Design review of the part built by this model. Coordinates are the model's own, in mm. Coordinates: 2 decimals unless noted, no trailing zeros. Order: outer loops, then holes, each group sorted by start corner. A loop starts at its lowest first (then second) coordinate and runs counter-clockwise, first axis right, second up. Notation, with made-up numbers: M 50,83 L 63,83 A21 cw 63,97 Z; hole C 81.5,-37 d8. An arc over 180 degrees is marked long. Answer as a JSON object with one key per item and string values.
Autodesk Inventor part; units mm, degrees
ref_plane "YZ Plane" through (0, 0, 0) normal (1, 0, 0) x (0, 1, 0)
ref_plane "XZ Plane" through (0, 0, 0) normal (0, 1, 0) x (-1, 0, 0)
ref_plane "XY Plane" through (0, 0, 0) normal (0, 0, 1) x (1, 0, 0)
sketch "Sketch1" plane through (0, 0, 0) normal (1, 0, 0) x (0, 1, 0)
  line L0 (4.9868, 295.4813) -> (-299.8132, 295.4813)
  line L1 (-299.8132, 295.4813) -> (-299.8132, -9.3187)
  line L2 (-299.8132, -9.3187) -> (4.9868, -9.3187)
  line L3 (4.9868, -9.3187) -> (4.9868, 295.4813)
  point P0 (0, 0)
  dimension "d0" = 304.8
  dimension "d1" = 304.8
extrude "Extrusion1" add sketch "Sketch1" along normal blind 3.175
sketch "Sketch2" plane through (3.175, 0, 0) normal (1, 0, 0) x (0, 0, -1)
  line L0 (-143.0813, 4.9868) -> (-143.0813, -147.4132)
  circle A0 centre (-143.0813, -147.4132) radius 12.7
  point P0 (0, 0)
  point P1 (9.3187, 4.9868)
  dimension "d4" = 152.4
  dimension "d5" = 25.4
extrude "Extrusion2" cut sketch "Sketch2" against normal blind 50.8
sketch "Sketch3" plane through (3.175, 0, 0) normal (1, 0, 0) x (0, 0, -1)
  circle A0 centre (-143.0813, -147.4132) radius 12.7
  circle A1 centre (-143.0813, -122.0132) radius 3.175
  circle A2 centre (-143.0813, -96.6132) radius 3.175
  circle A3 centre (-143.0813, -71.2132) radius 3.175
  circle A4 centre (-143.0813, -45.8132) radius 3.175
  circle A5 centre (-143.0813, -20.4132) radius 3.175
  circle A6 centre (-143.0813, 4.9868) radius 3.175
  line L0 (9.3187, -299.8132) -> (9.3187, 4.9868)
  circle A7 centre (-143.0813, -172.8132) radius 3.175
  circle A8 centre (-143.0813, -198.2132) radius 3.175
  circle A9 centre (-143.0813, -249.0132) radius 3.175
  circle A10 centre (-143.0813, -223.6132) radius 3.175
  circle A11 centre (-143.0813, -299.8132) radius 3.175
  circle A12 centre (-143.0813, -274.4132) radius 3.175
  circle A13 centre (-168.4813, -122.0132) radius 3.175
  circle A14 centre (-168.4813, -96.6132) radius 3.175
  circle A15 centre (-168.4813, -45.8132) radius 3.175
  circle A16 centre (-168.4813, -71.2132) radius 3.175
  circle A17 centre (-168.4813, 4.9868) radius 3.175
  circle A18 centre (-168.4813, -20.4132) radius 3.175
  circle A19 centre (-168.4813, -299.8132) radius 3.175
  circle A20 centre (-168.4813, -249.0132) radius 3.175
  circle A21 centre (-168.4813, -274.4132) radius 3.175
  circle A22 centre (-168.4813, -223.6132) radius 3.175
  circle A23 centre (-168.4813, -198.2132) radius 3.175
  circle A24 centre (-168.4813, -172.8132) radius 3.175
  circle A25 centre (-117.6813, -122.0132) radius 3.175
  circle A26 centre (-117.6813, -96.6132) radius 3.175
  circle A27 centre (-117.6813, -45.8132) radius 3.175
  circle A28 centre (-117.6813, -71.2132) radius 3.175
  circle A29 centre (-117.6813, 4.9868) radius 3.175
  circle A30 centre (-117.6813, -20.4132) radius 3.175
  circle A31 centre (-117.6813, -299.8132) radius 3.175
  circle A32 centre (-117.6813, -249.0132) radius 3.175
  circle A33 centre (-117.6813, -274.4132) radius 3.175
  circle A34 centre (-117.6813, -223.6132) radius 3.175
  circle A35 centre (-117.6813, -198.2132) radius 3.175
  circle A36 centre (-117.6813, -172.8132) radius 3.175
  circle A37 centre (-193.8813, -122.0132) radius 3.175
  circle A38 centre (-193.8813, -96.6132) radius 3.175
  circle A39 centre (-193.8813, -45.8132) radius 3.175
  circle A40 centre (-193.8813, -71.2132) radius 3.175
  circle A41 centre (-193.8813, 4.9868) radius 3.175
  circle A42 centre (-193.8813, -20.4132) radius 3.175
  circle A43 centre (-193.8813, -299.8132) radius 3.175
  circle A44 centre (-193.8813, -249.0132) radius 3.175
  circle A45 centre (-193.8813, -274.4132) radius 3.175
  circle A46 centre (-193.8813, -223.6132) radius 3.175
  circle A47 centre (-193.8813, -198.2132) radius 3.175
  circle A48 centre (-193.8813, -172.8132) radius 3.175
  circle A49 centre (-92.2813, -122.0132) radius 3.175
  circle A50 centre (-92.2813, -96.6132) radius 3.175
  circle A51 centre (-92.2813, -45.8132) radius 3.175
  circle A52 centre (-92.2813, -71.2132) radius 3.175
  circle A53 centre (-92.2813, 4.9868) radius 3.175
  circle A54 centre (-92.2813, -20.4132) radius 3.175
  circle A55 centre (-92.2813, -299.8132) radius 3.175
  circle A56 centre (-92.2813, -249.0132) radius 3.175
  circle A57 centre (-92.2813, -274.4132) radius 3.175
  circle A58 centre (-92.2813, -223.6132) radius 3.175
  circle A59 centre (-92.2813, -198.2132) radius 3.175
  circle A60 centre (-92.2813, -172.8132) radius 3.175
  point P0 (0, 0)
  dimension "d9" = 6.35
  dimension "d11" = 6.35
  dimension "d12" = 6.35
  dimension "d13" = 6.35
  dimension "d14" = 6.35
  dimension "d15" = 6.35
  dimension "d18" = 6.35
  dimension "d19" = 6.35
  dimension "d20" = 6.35
  dimension "d21" = 6.35
  dimension "d22" = 6.35
  dimension "d23" = 6.35
  dimension "d24" = 6.35
  dimension "d25" = 6.35
  dimension "d26" = 6.35
  dimension "d27" = 6.35
  dimension "d28" = 6.35
  dimension "d29" = 6.35
  dimension "d33" = 6.35
  dimension "d35" = 6.35
  dimension "d36" = 6.35
  dimension "d37" = 6.35
  dimension "d38" = 6.35
  dimension "d39" = 6.35
  dimension "d41" = 6.35
  dimension "d43" = 6.35
  dimension "d44" = 6.35
  dimension "d45" = 6.35
  dimension "d46" = 6.35
  dimension "d47" = 6.35
extrude "Extrusion3" cut sketch "Sketch3" against normal blind 50.8
sketch "Sketch4" plane through (3.175, 0, 0) normal (1, 0, 0) x (0, 0, -1)
  circle A0 centre (-143.0813, -147.4132) radius 12.7
  line L0 (-143.0813, -147.4132) -> (-117.6813, -147.4132)
  line L1 (-117.6813, -147.4132) -> (-92.2813, -147.4132)
  circle A1 centre (-92.2813, -147.4132) radius 3.175
  circle A2 centre (-117.6813, -147.4132) radius 3.175
  circle A3 centre (-193.8813, -147.4132) radius 3.175
  circle A4 centre (-168.4813, -147.4132) radius 3.175
  point P0 (0, 0)
  dimension "d54" = 25.4
  dimension "d55" = 25.4
  dimension "d56" = 6.35
  dimension "d57" = 6.35
extrude "Extrusion4" cut sketch "Sketch4" against normal blind 50.8 contours A1 | A2 L1 L0 | L0 L1 A2 | A3 | A4
sketch "Sketch5" plane through (3.175, 0, 0) normal (1, 0, 0) x (0, 0, -1)
  line L0 (-295.4813, 4.9868) -> (-295.4813, -299.8132)
  circle A0 centre (-244.6813, -249.0132) radius 7.9375
  circle A1 centre (-41.4813, -249.0132) radius 7.9375
  line L1 (-244.6813, -249.0132) -> (-244.6813, -45.8132) construction
  circle A2 centre (-244.6813, -45.8132) radius 7.9375
  circle A3 centre (-41.4813, -45.8132) radius 7.9375
  point P0 (0, 0)
  dimension "d63" = 15.875
  dimension "d67" = 203.2
  dimension "d69" = 15.875
  dimension "d70" = 15.875
extrude "Extrusion5" cut sketch "Sketch5" against normal blind 914.4
properties part number "Drill Jig Base"
1) To check wall thickness, follow L1, parallel to Y at x = 2, z = 244 (3 decimals); L2, parallel to Y at x = 1.1, z = 240; L3, parallel to Z at x = 1.3, y = -97. State the ranges of each line that lie inside material, in increasing order.
Taken from the geometry:
{"L1": "y = -299.813 to -256.921, -241.105 to -53.721, -37.905 to 4.987", "L2": "y = -299.81 to -255.42, -242.6 to -52.22, -39.4 to 4.99", "L3": "z = -9.32 to 89.13, 95.43 to 114.53, 120.83 to 139.93, 146.23 to 165.33, 171.63 to 190.73, 197.03 to 295.48"}
2) Add section A-A (z = 152). State the section outline as (x, y) points (3 decimals), and give its area (3 significant figures).
Taken from the geometry:
{"outline": "M 0,-299.813 L 3.175,-299.813 L 3.175,-156.455 L 0,-156.455 Z; M 0,-138.372 L 3.175,-138.372 L 3.175,4.987 L 0,4.987 Z", "area": "910 mm2"}
3) Add section B-B (z = 41). State the section outline as (x, y) points (3 decimals).
Taken from the geometry:
{"outline": "M 0,-299.813 L 3.175,-299.813 L 3.175,-256.936 L 0,-256.936 Z; M 0,-241.09 L 3.175,-241.09 L 3.175,-53.736 L 0,-53.736 Z; M 0,-37.89 L 3.175,-37.89 L 3.175,4.987 L 0,4.987 Z"}
4) Add section C-C (x = 0.8). Count the separate pieces of the cut face and the enclosed holes in it, and give its area (3 significant figures).
Taken from the geometry:
{"separate pieces": "1", "enclosed holes": "59", "area": "89,700 mm2"}
5) Insertion check: pin 1 Ø10 at (y, z) = (-249.01, 168.48) entering from +X (3 decimals). The pin has a flat end and moves straight along its axis. Give the tip position at first contact, or say it passes through.
Taken from the geometry:
{"pin 1": "stops at x = 3.175"}
6) Mouldability with a two-part tool opening along Z and no side actions: class faces 1 (the flat face through (0, -150, 179)), 2 (the cylindrical face through (1.61, -246.63, 237.11)) as released by +Z, released by -Z, zero draft, split by the parting line, or undercut.
Taken from the geometry:
{"face 1": "zero draft", "face 2": "undercut"}
